Verification items for the finished model (mm, model axes). Face numbers are marked on the shaded views. A direction names the side the tool comes from. Round coordinates to 2 decimals unless told otherwise and drop trailing zeros. Order: outer loops, then holes, each group sorted by start corner. A loop starts at its lowest first (then second) coordinate and runs counter-clockwise, first axis right, second up. Notation, with made-up numbers: (52, 54.5) -> (109, 54.5) arc R12 ccw to (109, 66.5) -> close; hole circle Ø2 at (-14, -5). An arc over 180 degrees is marked (long way). Write item = value, one per line. Start each with the question number.
from build123d import *

# Parameters (mm, degrees)
F1_DEPTH = 25
F2_DEPTH = 25
F3_DEPTH = 25
F4_DEPTH = 25


with BuildPart() as f1:
    # F0 (on Top) → F1 (new body)
    with BuildSketch(Plane.XY):
        Polygon((-128.336711, 467.34343), (-228.336711, 467.34343), (-280.336711, 375.412752), (-380.336711, 375.412752), (-380.336711, 275.412752), (-228.336711, 275.412752), (-228.336711, -12.65657), (-128.336711, -12.65657), align=None)
    extrude(amount=F1_DEPTH)

    # F0 (on Top) → F2 (join)
    with BuildSketch(Plane.XY):
        Polygon((-128.336711, 467.34343), (-228.336711, 467.34343), (-280.336711, 375.412752), (-380.336711, 375.412752), (-380.336711, 275.412752), (-228.336711, 275.412752), (-228.336711, -12.65657), (-128.336711, -12.65657), align=None)
    extrude(amount=F2_DEPTH)

    # F0 (on Top) → F3 (join)
    with BuildSketch(Plane.XY):
        Polygon((-128.336711, 467.34343), (-228.336711, 467.34343), (-280.336711, 375.412752), (-380.336711, 375.412752), (-380.336711, 275.412752), (-228.336711, 275.412752), (-228.336711, -12.65657), (-128.336711, -12.65657), align=None)
    extrude(amount=F3_DEPTH)

    # F0 (on Top) → F4 (join)
    with BuildSketch(Plane.XY):
        Polygon((-128.336711, 467.34343), (-228.336711, 467.34343), (-280.336711, 375.412752), (-380.336711, 375.412752), (-380.336711, 275.412752), (-228.336711, 275.412752), (-228.336711, -12.65657), (-128.336711, -12.65657), align=None)
    extrude(amount=F4_DEPTH)


solid = f1.part
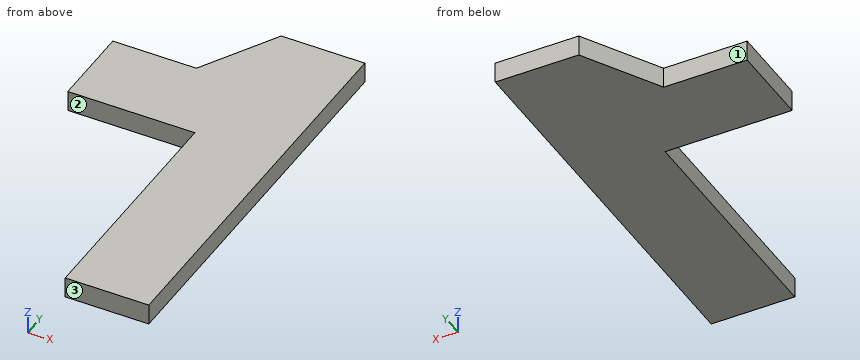
(1) Set-up check for the marked faces 1, 2 and 3: record each of +Z, -Z, +X, -X, +Y, -Y from which the full face is reachable in a straight line by a thin tool's end or side.
(2) Depth check by flat-ended pin: pin 1 (7.5 mm diameter, centred on x = -305.5, z = 17, fed in from -Y); pin 2 (7.5 mm diameter, centred on x = -344.5, z = 15.5, fed in from +Y). Enter the tip coordinate at first touch or a pass-through.
(3) Cross-section at C-C (y = 261). Enter the section's corners in (x, z).
(4) Cross-section at A-A (z = 11.5). Enter the section's corners in (x, y).
(5) Scan lines: line 1 along X through (y, z) = (150, 18.5); line 2 along Y through (x, z) = (-343.5, 18.5); line 3 along Y through (x, z) = (-266, 11.25). Record each from-to range of solid material in increasing order. Write a range as from..to.
(6) Cross-section at B-B (x = -349). Enter the section's corners in (y, z), and give its area (3 significant figures).
Outcome:
q1.face_1 = +Z, -Z, -X, +Y
q1.face_2 = +Z, -Z, -X, -Y
q1.face_3 = +Z, -Z, +X, -X, -Y
q2.pin_1 = 275.41
q2.pin_2 = 375.41
q3.outline = (-228.34, 0) -> (-128.34, 0) -> (-128.34, 25) -> (-228.34, 25) -> close
q4.outline = (-380.34, 275.41) -> (-228.34, 275.41) -> (-228.34, -12.66) -> (-128.34, -12.66) -> (-128.34, 467.34) -> (-228.34, 467.34) -> (-280.34, 375.41) -> (-380.34, 375.41) -> close
q5.line_1 = -228.34..-128.34
q5.line_2 = 275.41..375.41
q5.line_3 = 275.41..400.76
q6.outline = (275.41, 0) -> (375.41, 0) -> (375.41, 25) -> (275.41, 25) -> close
q6.area = 2,500 mm^2
